Read the model definition and answer for the solid it produces. Units are mm, in the model's axes. Face numbers are marked on the shaded views. Give positions to 0.01 mm unless a question says otherwise; leave off trailing zeros. Order: outer loops, then holes, each group sorted by start corner. A loop starts at its lowest first (then second) coordinate and runs counter-clockwise, first axis right, second up. Notation, with made-up numbers: (-14, 82.25) -> (0, 82.25) arc R17 cw to (0, 88.25) -> close; hole circle Ø8 at (-20, 47). An arc over 180 degrees is marked (long way). Answer as CSV lines item,"result". Start each with the question number.
1) A flat-ended cylindrical pin translates along its axis: pin 1 Ø3 at (x, z) = (0, 6.35) entering from -Y. Find the tip coordinate at first contact, or state that the pin passes through.
2) The mould has two halves that part along Z. Classify the marked faces 1, 2 and 3: +Z half, -Z half, draft (parallel to the pull), parting line (faces both ways), or undercut.
3) Straight lines are drawn through the part: L1, parallel to Z at x = 0, y = 1.75 (3 decimals); L2, parallel to X at y = 1, z = -6.35; L3, parallel to X at y = -0.25, z = 5.75. For each, find the intervals that lie inside material, in ascending order. Write a range as from..to.
4) Find section A-A (z = -6.35). Determine the outline of the cut face in (x, y) (3 decimals).
5) Find section D-D (z = 7.75). Determine the outline of the cut face in (x, y) (3 decimals).
6) Find section C-C (y = 0.5). Determine the outline of the cut face in (x, z) (3 decimals).
7) Find section B-B (x = 0). Determine the outline of the cut face in (y, z) (3 decimals).
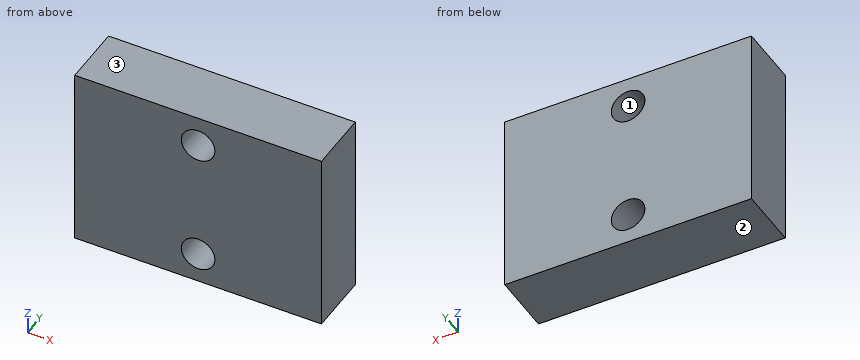
```python
from build123d import *

# Parameters (mm, degrees)
SKETCH1_W             = 25.4
SKETCH1_H             = 19.05
BOSS_EXTRUDE1_DEPTH   = 3.175
F_8_32_TAPPED_HOLE1_D = 3.4544


with BuildPart() as part:
    # Sketch1 → Boss-Extrude1 (new, symmetric)
    with BuildSketch(Plane(origin=(0, 0, 0), x_dir=(1, 0, 0), z_dir=(0, 1, 0))):
        Rectangle(SKETCH1_W, SKETCH1_H)
    extrude(amount=BOSS_EXTRUDE1_DEPTH, both=True)

    # #8-32 Tapped Hole1 (through all)
    with Locations(Plane(origin=(0, 3.175, 0), x_dir=(1, 0, 0), z_dir=(0, 1, 0))):
        with Locations((0, 6.35), (0, -6.35)):
            Hole(F_8_32_TAPPED_HOLE1_D / 2)


solid = part.part
```
Findings below:
1,pin 1,"through"
2,face 1,"undercut"
2,face 2,"-Z half"
2,face 3,"+Z half"
3,L1,"-9.525..-8.077, -4.623..4.623, 8.077..9.525"
3,L2,"-12.7..-1.73, 1.73..12.7"
3,L3,"-12.7..-1.62, 1.62..12.7"
4,outline,"(-12.7, -3.175) -> (-1.727, -3.175) -> (-1.727, 3.175) -> (-12.7, 3.175) -> close; (1.727, -3.175) -> (12.7, -3.175) -> (12.7, 3.175) -> (1.727, 3.175) -> close"
5,outline,"(-12.7, -3.175) -> (-1.012, -3.175) -> (-1.012, 3.175) -> (-12.7, 3.175) -> close; (1.012, -3.175) -> (12.7, -3.175) -> (12.7, 3.175) -> (1.012, 3.175) -> close"
6,outline,"(-12.7, -9.525) -> (12.7, -9.525) -> (12.7, 9.525) -> (-12.7, 9.525) -> close; hole circle Ø3.454 at (0, -6.35); hole circle Ø3.454 at (0, 6.35)"
7,outline,"(-3.175, -9.525) -> (3.175, -9.525) -> (3.175, -8.077) -> (-3.175, -8.077) -> close; (-3.175, -4.623) -> (3.175, -4.623) -> (3.175, 4.623) -> (-3.175, 4.623) -> close; (-3.175, 8.077) -> (3.175, 8.077) -> (3.175, 9.525) -> (-3.175, 9.525) -> close"
